Answer from the drawing. Dimensions are ordinates in mm from the lowest x, y and z of the part. A direction names the side the tool comes from. Round coordinates to 2 decimals unless told otherwise and drop trailing zeros. Order: outer loops, then holes, each group sorted by start corner. A loop starts at its lowest first (then second) coordinate and runs counter-clockwise, first axis right, second up. Notation, with made-up numbers: (49, 0) -> (76, 0) arc R20 ccw to (76, 32) -> close; hole circle Ø5 at (41.5, 17.5). An arc over 180 degrees is marked (long way). Use a Markdown table: item, result. Add a question column.
Item 1: A cutting plane is placed at A-A, the plane x = 2.75. Determine the outline of the cut face in (y, z), plus the area to 3 significant figures.
Item 2: A tool of negligible diameter and unlimited length cuts with its end or side. For the marked faces 4, 5 and 6, from which of +Z, -Z, +X, -X, +Y, -Y can it reach the whole face along a straight path? Write none if from no direction.
Item 3: A cutting plane is placed at B-B, the plane z = 8.5. Determine the outline of the cut face in (x, y).
Item 4: A cutting plane is placed at C-C, the plane y = 14.25. Determine the outline of the cut face in (x, z), plus the area to 3 significant figures.
Item 5: Flat-ended cylindrical pins translate along their axes: P1, Ø1, axis at x = 4.5, z = 3, coming from the -Y side; P2, Ø5.5, axis at x = 11, y = 3, coming from the +Z side; P3, Ø4, axis at x = 8, y = 15, coming from the -Z side; P4, Ø2.5, axis at x = 9, z = 8.5, coming from the -Y side. Find the tip coordinate at first contact, or state that the pin passes through.
Item 6: For a pull along Z with two mould halves and no side action, classify the marked faces 1, 2 and 3 as +Z half, -Z half, draft (parallel to the pull), parting line (faces both ways), or undercut.
Item 7: Find the intervals of material crossed by L1, parallel to Y at x = 3, z = 7.25; L2, parallel to Y at x = 8.75, z = 3.5; L3, parallel to Z at x = 12, y = 6.75, in increasing order. Write a range as [from, to].
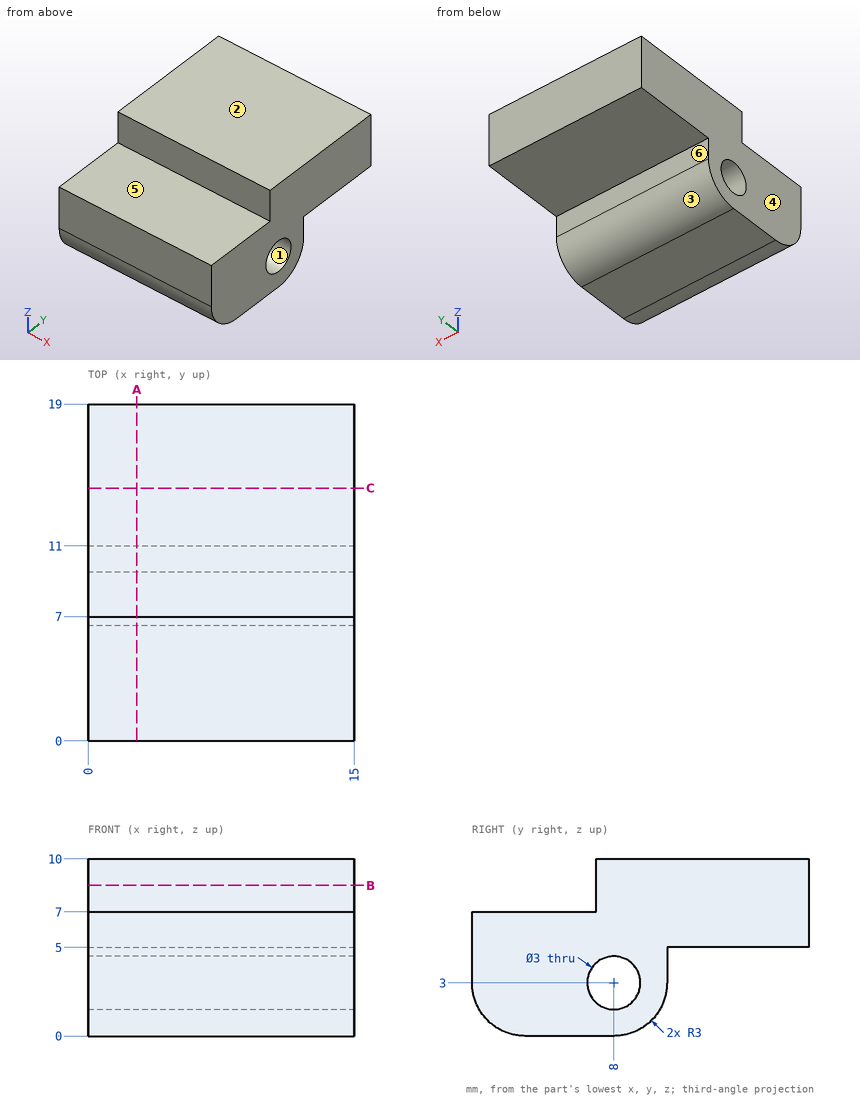
Reported:
| question | item | result |
|---|---|---|
| 1 | outline | (0, 3) arc R3 ccw to (3, 0) -> (8, 0) arc R3 ccw to (11, 3) -> (11, 5) -> (19, 5) -> (19, 10) -> (7, 10) -> (7, 7) -> (0, 7) -> close; hole circle Ø3 at (8, 3) |
| 1 | area | 118 mm² |
| 2 | face 4 | +Z, -Z, -X, +Y, -Y |
| 2 | face 5 | +Z, +X, -X, -Y |
| 2 | face 6 | -Z, +X, -X, +Y |
| 3 | outline | (0, 7) -> (15, 7) -> (15, 19) -> (0, 19) -> close |
| 4 | outline | (0, 5) -> (15, 5) -> (15, 10) -> (0, 10) -> close |
| 4 | area | 75.0 mm² |
| 5 | P1 | y = 0 |
| 5 | P2 | z = 7 |
| 5 | P3 | z = 5 |
| 5 | P4 | y = 7 |
| 6 | face 1 | undercut |
| 6 | face 2 | +Z half |
| 6 | face 3 | -Z half |
| 7 | L1 | [7, 19] |
| 7 | L2 | [0, 6.59], [9.41, 11] |
| 7 | L3 | [0, 2.17], [3.83, 7] |
